```python
from build123d import *

# Parameters (mm, degrees)
EXTRUDE_START       = -15
SKETCH_1_R          = 12.5
EXTRUDE_1_DEPTH     = 55
SKETCH_2_W          = 7.63538833
SKETCH_2_H          = 30
CUT_EXTRUDE_2_DEPTH = 25
FILLET_1_R          = 3
SKETCH_3_R          = 4
CUT_EXTRUDE_3_DEPTH = 25
FILLET_2_R          = 3


with BuildPart() as part:
    # Эскиз1 → Вытянуть1 (new body)
    with BuildSketch(Plane(origin=(0, 0, 0), x_dir=(1, 0, 0), z_dir=(0, 1, 0)).offset(EXTRUDE_START)):
        with Locations(Location((0, 0, 0), (0, 0, 270))):
            Circle(SKETCH_1_R)
    extrude(amount=EXTRUDE_1_DEPTH)

    # Эскиз2 → Вытянуть2 (cut, symmetric)
    with BuildSketch(Plane(origin=(0, 0, 0), x_dir=(0, 0, -1), z_dir=(1, 0, 0))):
        Rectangle(SKETCH_2_W, SKETCH_2_H)
    extrude(amount=CUT_EXTRUDE_2_DEPTH, both=True, mode=Mode.SUBTRACT)

    # Скругление1
    fillet_1_edges = [part.edges().sort_by_distance(p)[0] for p in [
        (0, -15, -12.5),
        (7.366438181, -15, 10.098791439),
    ]]
    fillet(fillet_1_edges, radius=FILLET_1_R)

    # Эскиз3 → Вытянуть3 (cut, symmetric)
    with BuildSketch(Plane.XY):
        with Locations((0, -4.581717599)):
            Circle(SKETCH_3_R)
    extrude(amount=CUT_EXTRUDE_3_DEPTH, both=True, mode=Mode.SUBTRACT)

    # Скругление2
    fillet_2_edges = [part.edges().sort_by_distance(p)[0] for p in [
        (0, 15, -3.817694165),
        (0, 15, 3.817694165),
    ]]
    fillet(fillet_2_edges, radius=FILLET_2_R)


solid = part.part
```
For this review, take the finished solid that the model builds, in its own axes (mm). A direction names the side the tool comes from. Round coordinates to 2 decimals unless told otherwise and drop trailing zeros. Order: outer loops, then holes, each group sorted by start corner. A loop starts at its lowest first (then second) coordinate and runs counter-clockwise, first axis right, second up.
Q1. We need section D-D, the plane y = 17. Give the boundary of the cut face in (x, z).
Findings below:
outline: circle Ø25 at (0, 0)
Q2. We need section A-A, the plane x = 0. Give the boundary of the cut face in (y, z), plus the area to 3 significant figures.
Findings below:
outline: (-15, -9.5) arc R3 ccw to (-12, -12.5) - (-8.58, -12.5) - (-8.58, -3.82) - (-15, -3.82) - close; (-15, 3.82) - (-8.58, 3.82) - (-8.58, 12.5) - (-12, 12.5) arc R3 ccw to (-15, 9.5) - close; (-0.58, -12.5) - (40, -12.5) - (40, 12.5) - (-0.58, 12.5) - (-0.58, 3.82) - (12, 3.82) arc R3 cw to (15, 0.82) - (15, -0.82) arc R3 cw to (12, -3.82) - (-0.58, -3.82) - close
area: 1,010 mm2
Q3. We need section B-B, the plane y = 10. Give the boundary of the cut face in (x, z), plus the area to 3 significant figures.
Findings below:
outline: (-11.9, -3.82) arc R12.5 ccw to (11.9, -3.82) - close; (-11.9, 3.82) - (11.9, 3.82) arc R12.5 ccw to start
area: 303 mm2
Q4. Machinability: for faces 1 (the flat face through (0, 40, 0)), 2 (the flat face through (0, 1, 3.818)), which of the approach directions +Z, -Z, +X, -X, +Y, -Y give a long, thin tool a straight path to every point of the face, cutting with its end or side? Answer none if there is none.
Findings below:
face 1: +Z, -Z, +X, -X, +Y
face 2: +X, -X, -Y
Q5. Mouldability with a two-part tool opening along X and no side actions: class faces 3 (the cylindrical face through (-4.788, 13.636, 11.547)), 4 (the cylindrical face through (-3.996, -4.406, 8.22)), 5 (the flat face through (0, 15, 0)), 6 (the cylindrical face through (-3.996, -4.406, -8.098)) as pulls with the +X half, pulls with the -X half, needs draft (parallel to the pull), parting line crosses it, or undercut.
Findings below:
face 3: parting line crosses it
face 4: undercut
face 5: needs draft
face 6: undercut
Q6. We need section C-C, the plane z = 0. Give the boundary of the cut face in (x, y), plus the area to 3 significant figures.
Findings below:
outline: (-12.5, 15) - (12.5, 15) - (12.5, 40) - (-12.5, 40) - close
area: 625 mm2
Q7. Insertion check: P1, Ø3, axis at y = 11.5, z = 3.5, coming from the +X side; P2, Ø4, axis at y = 26, z = 8, coming from the -X side; P3, Ø1, axis at x = 8.5, z = 2, coming from the -Y side; P4, Ø3, axis at x = -1.5, y = 14.5, coming from the +Z side. Each pin has a flat end and moves straight along its axis. Give the tip position at first contact, or say it passes through.
Findings below:
P1: stops at x = 11.96
P2: stops at x = -10.97
P3: stops at y = 14.48
P4: stops at z = 12.5
Q8. Wall thickness on line 1 (Y direction, x = 0, z = -8.5); line 2 (X direction, y = 32, z = 0); line 3 (Y direction, x = -1.5, z = -7.75): over which ranges is each line inside the solid? List them lowest first.
Findings below:
line 1: y = -15 to -8.58, -0.58 to 40
line 2: x = -12.5 to 12.5
line 3: y = -15 to -8.29, -0.87 to 40
